```python
from build123d import *

# Parameters (mm, degrees)
F0_W     = 485.775
F0_H     = 19.05
F0_R     = 1.5875
F0_H_2   = 127
F1_DEPTH = 9.525
F0_H_3   = 9.525
F2_DEPTH = 9.525
F4_R     = 1.5875
F5_DEPTH = 9.525
F3_R     = 1.5875
F6_DEPTH = 9.525


with BuildPart() as f1:
    # F0 (on Right) → F1 (new body)
    with BuildSketch(Plane.YZ):
        with Locations((0, -148.74875)):
            Rectangle(F0_W, F0_H)
        with Locations((-230.1875, -148.74875)):
            Circle(F0_R, mode=Mode.SUBTRACT)
        with Locations((-88.9, -148.74875)):
            Circle(F0_R, mode=Mode.SUBTRACT)
        with Locations((86.36, -148.74875)):
            Circle(F0_R, mode=Mode.SUBTRACT)
        with Locations((230.1875, -148.74875)):
            Circle(F0_R, mode=Mode.SUBTRACT)
        with Locations((0, -75.72375)):
            Rectangle(F0_W, F0_H_2)
        with BuildLine():
            Line((-50.8, -101.12375), (50.8, -101.12375))
            ThreePointArc((50.8, -101.12375), (57.15, -107.47375), (50.8, -113.82375))
            Line((50.8, -113.82375), (-50.8, -113.82375))
            ThreePointArc((-50.8, -113.82375), (-57.15, -107.47375), (-50.8, -101.12375))
        make_face(mode=Mode.SUBTRACT)
        with BuildLine():
            ThreePointArc((50.8, -113.82375), (57.15, -107.47375), (50.8, -101.12375))
            Line((50.8, -101.12375), (-50.8, -101.12375))
            ThreePointArc((-50.8, -101.12375), (-57.15, -107.47375), (-50.8, -113.82375))
            Line((-50.8, -113.82375), (50.8, -113.82375))
        make_face()
    extrude(amount=F1_DEPTH)

    # F0 (on Right) → F2 (join)
    with BuildSketch(Plane.YZ):
        with Locations((0, -75.72375)):
            Rectangle(F0_W, F0_H_2)
        with BuildLine():
            Line((-50.8, -101.12375), (50.8, -101.12375))
            ThreePointArc((50.8, -101.12375), (57.15, -107.47375), (50.8, -113.82375))
            Line((50.8, -113.82375), (-50.8, -113.82375))
            ThreePointArc((-50.8, -113.82375), (-57.15, -107.47375), (-50.8, -101.12375))
        make_face(mode=Mode.SUBTRACT)
        with Locations((0, -7.46125)):
            Rectangle(F0_W, F0_H_3)
        with BuildLine():
            ThreePointArc((50.8, -113.82375), (57.15, -107.47375), (50.8, -101.12375))
            Line((50.8, -101.12375), (-50.8, -101.12375))
            ThreePointArc((-50.8, -101.12375), (-57.15, -107.47375), (-50.8, -113.82375))
            Line((-50.8, -113.82375), (50.8, -113.82375))
        make_face()
    extrude(amount=-F2_DEPTH)

    # F4 (on face) → F5 (cut)
    with BuildSketch(Plane(origin=(0, 242.8875, 0), x_dir=(-1, 0, 0), z_dir=(0, 1, 0))):
        with Locations((0, -43.97375)):
            Circle(F4_R)
        with Locations((0, -113.82375)):
            Circle(F4_R)
    extrude(amount=-F5_DEPTH, mode=Mode.SUBTRACT)

    # F3 (on face) → F6 (cut)
    with BuildSketch(Plane.XZ.offset(242.8875)):
        with Locations((0, -113.82375)):
            Circle(F3_R)
        with Locations((0, -43.97375)):
            Circle(F3_R)
    extrude(amount=-F6_DEPTH, mode=Mode.SUBTRACT)


solid = f1.part
```
Verification items for the finished model (mm, model axes). A direction names the side the tool comes from. Coordinates: 2 decimals unless noted, no trailing zeros. Loops run counter-clockwise (first coordinate to the right, second up) from the corner with the lowest first, then second, coordinate; pieces in that order, holes last. Notation, with made-up numbers: (-15.75, 85) - (42.25, 85) arc R14 ccw to (42.25, 112) - close; hole circle Ø10 at (-35, 45.25). An arc over 180 degrees is marked (long way). Put each result on its own line as item: value.
Item 1: Section check B-B (x = 4.75). Enter the section's corners in (y, z) (1 decimal), then the cut area to 3 significant figures.
Conclusion:
outline: (-242.9, -158.3) - (242.9, -158.3) - (242.9, -12.2) - (-242.9, -12.2) - close; hole circle Ø3.2 at (-230.2, -148.7); hole circle Ø3.2 at (-88.9, -148.7); hole circle Ø3.2 at (86.4, -148.7); hole circle Ø3.2 at (230.2, -148.7)
area: 70,900 mm2
Item 2: Scan lines: line 1 along Z through (x, y) = (3.75, -88.9); line 2 along Z through (x, y) = (-7.75, 136); line 3 along Z through (x, y) = (6.5, 132.5). Record each from-to range of solid material in increasing order.
Conclusion:
line 1: z = -158.27 to -150.34, -147.16 to -12.22
line 2: z = -139.22 to -2.7
line 3: z = -158.27 to -12.22
Item 3: Set-up check for faces 1 (the face through (0, -3, -149)), 2 (the face through (0, -3, -7)), 3 (the face through (5, -3, -158.274)): record each of +Z, -Z, +X, -X, +Y, -Y from which the full face is reachable in a straight line by a thin tool's end or side.
Conclusion:
face 1: -Z, -X, +Y, -Y
face 2: +Z, +X, +Y, -Y
face 3: -Z, +X, -X, +Y, -Y
Item 4: Section check A-A (y = -138). Enter the section's corners in (x, z) (3 decimals), then the cut area to 3 significant figures.
Conclusion:
outline: (-9.525, -139.224) - (0, -139.224) - (0, -158.274) - (9.525, -158.274) - (9.525, -12.224) - (0, -12.224) - (0, -2.699) - (-9.525, -2.699) - close
area: 2,690 mm2
Item 5: Gauge pin test, flat ends, axial feed: pin 1 Ø1.9 at (x, z) = (0, -113.82) entering from +Y; pin 2 Ø2 at (x, y) = (7.5, -140.5) entering from +Z; pin 3 Ø15 at (y, z) = (113.5, -152) entering from -X. Record the tip position at first contact, or that the pin passes through.
Conclusion:
pin 1: stops at y = 233.36
pin 2: stops at z = -12.22
pin 3: stops at x = 0
